Verification items for the finished model (mm, model axes). Face numbers are marked on the shaded views. A direction names the side the tool comes from. Round coordinates to 2 decimals unless told otherwise and drop trailing zeros. Write each loop counter-clockwise with the first axis right and the second up, starting at its lowest first coordinate (ties: lowest second). Pieces come first, ordered by that corner, then holes. Notation, with made-up numbers: (62.5, -16.5) - (91.5, -16.5) arc R18 ccw to (91.5, 6.5) - close; hole circle Ø7 at (14.25, -26). An arc over 180 degrees is marked (long way). Answer as a JSON object with one key per item and string values.
```python
from build123d import *

# Parameters (mm, degrees)
T_LE_DE_BASE_PLI_E1_DEPTH = 32
ESQUISSE6_R               = 4.5
ENL_V_MAT_EXTRU_1_DEPTH   = 10
ESQUISSE7_R               = 0.7
ENL_V_MAT_EXTRU_2_DEPTH   = 64.780874876


# Sheet-metal steps are written as plain solids
with BuildPart() as part:
    # Esquisse1 → Tôle de base pliée1 (new body)
    with BuildSketch(Plane.XY):
        with BuildLine():
            Line((-40, 19), (-3.7366, 19))
            ThreePointArc((-3.7366, 19), (-1.094424801, 17.905575199), (0, 15.2634))
            Line((0, 15.2634), (0, -15.2634))
            ThreePointArc((0, -15.2634), (-1.094424801, -17.905575199), (-3.7366, -19))
            Line((-3.7366, -19), (-40, -19))
            Line((-40, -19), (-40, -16))
            Line((-40, -16), (-3.7366, -16))
            ThreePointArc((-3.7366, -16), (-3.215745145, -15.784254855), (-3, -15.2634))
            Line((-3, -15.2634), (-3, 15.2634))
            ThreePointArc((-3, 15.2634), (-3.215745145, 15.784254855), (-3.7366, 16))
            Line((-3.7366, 16), (-40, 16))
            Line((-40, 16), (-40, 19))
        make_face()
    extrude(amount=T_LE_DE_BASE_PLI_E1_DEPTH)

    # Esquisse6 → Enlèv. mat.-Extru.1 (cut)
    with BuildSketch(Plane.XZ.offset(19)):
        with Locations((-10.7366, 16)):
            Circle(ESQUISSE6_R)
    extrude(amount=-ENL_V_MAT_EXTRU_1_DEPTH, mode=Mode.SUBTRACT)

    # Esquisse7 → Enlèv. mat.-Extru.2 (cut, through all)
    with BuildSketch(Plane(origin=(0, 19, 0), x_dir=(1, 0, 0), z_dir=(0, 1, 0))):
        with Locations(Location((-37, -29.5, 0), (0, 0, 270))):
            Circle(ESQUISSE7_R)
        with Locations(Location((-37, -2.5, 0), (0, 0, 270))):
            Circle(ESQUISSE7_R)
    extrude(amount=-ENL_V_MAT_EXTRU_2_DEPTH, mode=Mode.SUBTRACT)


solid = part.part
```
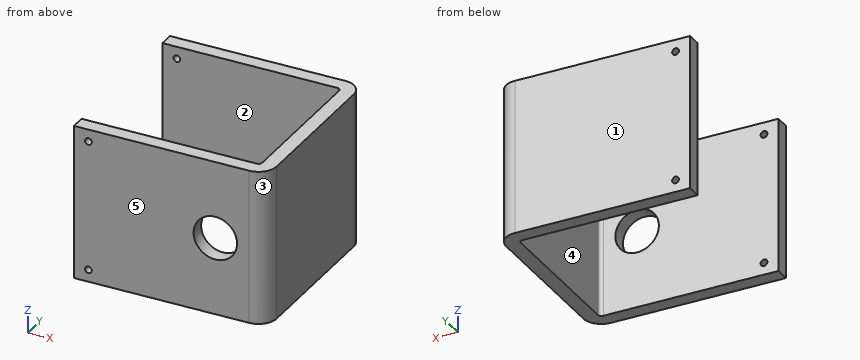
1. Go/stop test with a flat-tipped pin: pin 1 (1 mm diameter, centred on y = -7.5, z = 10.5, fed in from -X). Record where the tip stops, or that it passes through.
Completed:
{"pin 1": "stops at x = -3"}
2. Cross-section at A-A (z = 16). Record the boundary of the cut face in (x, y).
Completed:
{"outline": "(-40, -19) - (-15.24, -19) - (-15.24, -16) - (-40, -16) - close; (-40, 16) - (-3.74, 16) arc R0.74 cw to (-3, 15.26) - (-3, -15.26) arc R0.74 cw to (-3.74, -16) - (-6.24, -16) - (-6.24, -19) - (-3.74, -19) arc R3.74 ccw to (0, -15.26) - (0, 15.26) arc R3.74 ccw to (-3.74, 19) - (-40, 19) - close"}
3. Access from +Z, -Z, +X, -X, +Y, -Y to the whole of each face (thin tool, end or side, straight path). Record for the marked faces 4 and 5.
Completed:
{"face 4": "+Z, -Z, -X", "face 5": "+Z, -Z, +X, -X, -Y"}
4. Cross-section at C-C (z = 29.5). Record the boundary of the cut face in (x, y).
Completed:
{"outline": "(-40, -19) - (-37.7, -19) - (-37.7, -16) - (-40, -16) - close; (-40, 16) - (-37.7, 16) - (-37.7, 19) - (-40, 19) - close; (-36.3, -19) - (-3.74, -19) arc R3.74 ccw to (0, -15.26) - (0, 15.26) arc R3.74 ccw to (-3.74, 19) - (-36.3, 19) - (-36.3, 16) - (-3.74, 16) arc R0.74 cw to (-3, 15.26) - (-3, -15.26) arc R0.74 cw to (-3.74, -16) - (-36.3, -16) - close"}
5. Mould release check, pull along Y, two halves, no side actions. Record for the marked faces 1, 2 and 3: released by +Y, released by -Y, zero draft, split by the parting line, or undercut.
Completed:
{"face 1": "released by +Y", "face 2": "undercut", "face 3": "released by -Y"}
6. Cross-section at D-D (x = -11). Record the boundary of the cut face in (y, z).
Completed:
{"outline": "(-19, 0) - (-16, 0) - (-16, 11.51) - (-19, 11.51) - close; (-19, 20.49) - (-16, 20.49) - (-16, 32) - (-19, 32) - close; (16, 0) - (19, 0) - (19, 32) - (16, 32) - close"}
7. Cross-section at B-B (x = -33). Record the boundary of the cut face in (y, z), plus the area to 3 significant figures.
Completed:
{"outline": "(-19, 0) - (-16, 0) - (-16, 32) - (-19, 32) - close; (16, 0) - (19, 0) - (19, 32) - (16, 32) - close", "area": "192 mm^2"}
8. Material ranges on probe 1 along Z at (x, y) = (-37, 16.65); probe 2 along Y at (x, z) = (-15, 14); probe 3 along X at (y, z) = (-10, 30.5), recorded low to high. Write a range as from..to.
Completed:
{"probe 1": "z = 0..1.8, 3.2..28.8, 30.2..32", "probe 2": "y = -19..-16, 16..19", "probe 3": "x = -3..0"}
